Geometry check sheet. Reference: drawing and pictorial views, mm from the part's lowest x, y, z. A direction names the side the tool comes from. Give positions to 0.01 mm unless a question says otherwise; leave off trailing zeros. Loops run counter-clockwise (first coordinate to the right, second up) from the corner with the lowest first, then second, coordinate; pieces in that order, holes last. Notation, with made-up numbers: (48.5, 84) - (93.5, 84) arc R22 cw to (93.5, 121) - close; hole circle Ø2 at (-24.5, 8.25). An arc over 180 degrees is marked (long way). One line per question, with ' | ' between items. Start each with the question number.
1. Section check C-C, the plane z = 230. Enter the section's corners in (x, y).
2. Section check A-A, the plane y = 40. Enter the section's corners in (x, z), then the cut area to 3 significant figures.
3. Depth check by flat-ended pin: pin 1 Ø8 at (y, z) = (47, 141.5) entering from -X; pin 2 Ø4 at (y, z) = (28.5, 186) entering from -X; pin 3 Ø8 at (y, z) = (26.5, 218.5) entering from +X. Enter the tip coordinate at first touch or a pass-through.
4. Thickness scan on line 1 along X through (y, z) = (64, 294); line 2 along Z through (x, y) = (85.5, 66.5); line 3 along Z through (x, y) = (18.5, 22). Record the ranges inside material, lowest first. Write a range as from..to.
5. Tool access check on the marked faces 1, 2 and 3. Record the directions out of +Z, -Z, +X, -X, +Y, -Y that give a thin tool (end or side, any length) a straight path to the whole face; none if there is none.
6. Section check B-B, the plane x = 54. Enter the section's corners in (y, z), then the cut area to 3 significant figures.
7. Section check D-D, the plane y = 69.5. Enter the section's corners in (x, z).
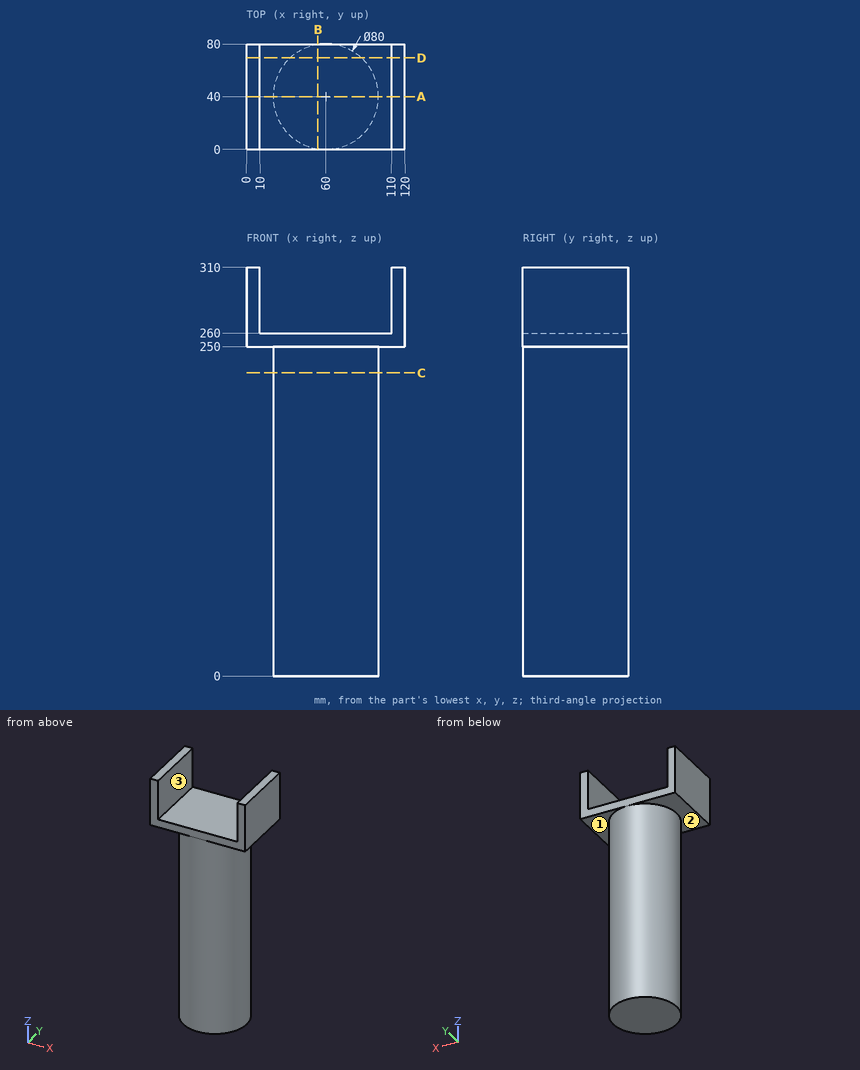
Results list:
1) outline: circle Ø80 at (60, 40)
2) outline: (0, 250) - (20, 250) - (20, 0) - (100, 0) - (100, 250) - (120, 250) - (120, 310) - (110, 310) - (110, 260) - (10, 260) - (10, 310) - (0, 310) - close | area: 22,200 mm²
3) pin 1: x = 20.11 | pin 2: x = 21.14 | pin 3: x = 98.86
4) line 1: 0..10, 110..120 | line 2: 0..260 | line 3: 250..260
5) face 1: -Z, +X | face 2: -Z, -X | face 3: +Z, +Y, -Y
6) outline: (0, 250) - (0.45, 250) - (0.45, 0) - (79.55, 0) - (79.55, 250) - (80, 250) - (80, 260) - (0, 260) - close | area: 20,600 mm²
7) outline: (0, 250) - (32.99, 250) - (32.99, 0) - (87.01, 0) - (87.01, 250) - (120, 250) - (120, 310) - (110, 310) - (110, 260) - (10, 260) - (10, 310) - (0, 310) - close
